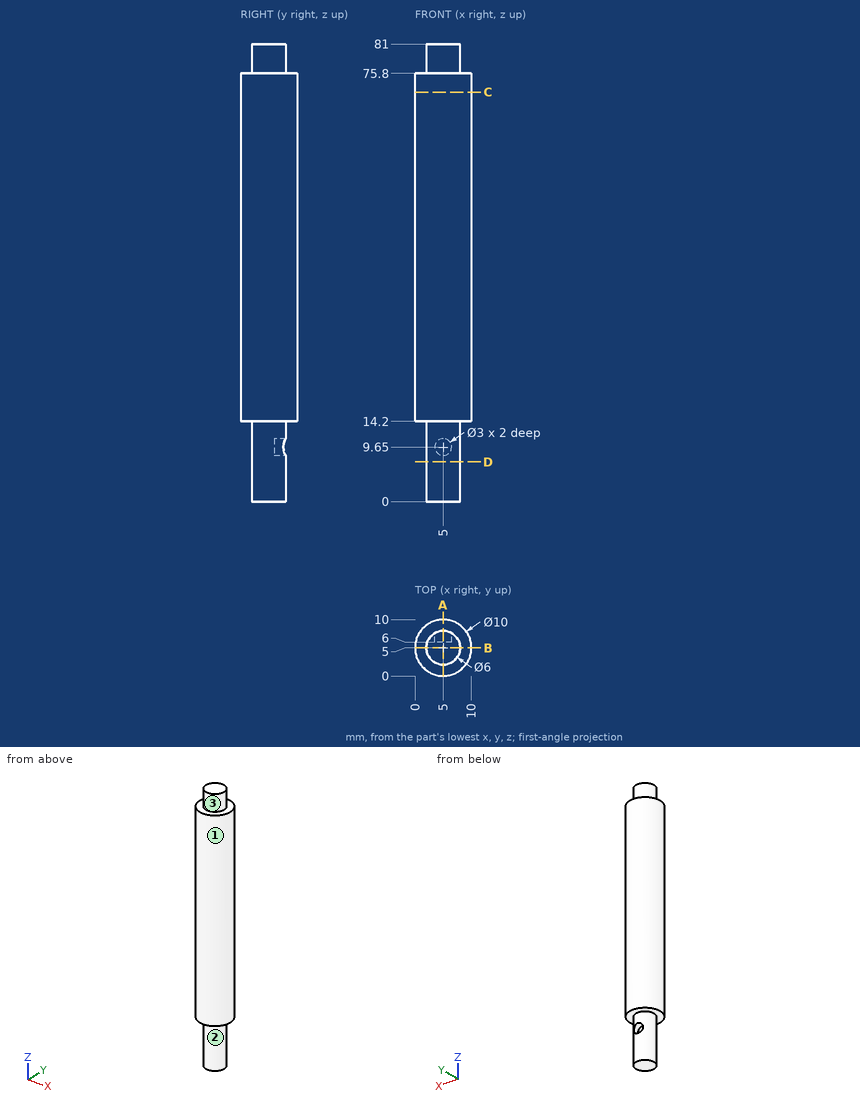
Can you work these out from the drawing? Everything is in mm from the part's minimum corner. A direction names the side the tool comes from. Round coordinates to 2 decimals unless told otherwise and drop trailing zeros. Order: outer loops, then holes, each group sorted by start corner. A loop starts at its lowest first (then second) coordinate and runs counter-clockwise, first axis right, second up. Notation, with made-up numbers: M 21,44 L 26,44 A29 ccw 26,77 Z; hole C 56,65 d9. An arc over 180 degrees is marked long. One line per question, with ' | ' between items.
1) I want a section at C-C, the plane z = 72.5. Write out the boundary of the cut face in (x, y), then the cut area to 3 significant figures.
Working result:
outline: C 5,5 d10 | area: 78.5 mm²
2) I want a section at B-B, the plane y = 5. Write out the boundary of the cut face in (x, z), then the cut area to 3 significant figures.
Working result:
outline: M 0,14.2 L 2,14.2 L 2,0 L 8,0 L 8,14.2 L 10,14.2 L 10,75.8 L 8,75.8 L 8,81 L 2,81 L 2,75.8 L 0,75.8 Z | area: 732 mm²
3) I need wall thicknesses on line 1 along Z through (x, y) = (5, 7.5); line 2 along X through (y, z) = (6.9, 9.65); line 3 along X through (y, z) = (7.2, 9.65). Which ranges of each line are inside material? Lowest first, please.
Working result:
line 1: 0 to 8.15, 11.15 to 81 | line 2: 2.68 to 3.5, 6.5 to 7.32 | line 3: 2.96 to 3.5, 6.5 to 7.04
4) I want a section at A-A, the plane x = 5. Write out the boundary of the cut face in (y, z), then the cut area to 3 significant figures.
Working result:
outline: M 0,14.2 L 2,14.2 L 2,0 L 8,0 L 8,8.15 L 6,8.15 L 6,11.15 L 8,11.15 L 8,14.2 L 10,14.2 L 10,75.8 L 8,75.8 L 8,81 L 2,81 L 2,75.8 L 0,75.8 Z | area: 726 mm²
5) I want a section at D-D, the plane z = 7. Write out the boundary of the cut face in (x, y), then the cut area to 3 significant figures.
Working result:
outline: C 5,5 d6 | area: 28.3 mm²
6) For pin 1 Ø1 at (x, z) = (6, 51.5) entering from +Y; pin 2 Ø5 at (x, z) = (3.5, 24.5) entering from -Y; pin 3 Ø2.5 at (x, z) = (4.5, 10) entering from +Y; pin 4 Ø1 at (y, z) = (6.5, 12.5) entering from -X, each with a flat end and sliding along its axis, tell me the tip position at first contact or that it passes through.
Working result:
pin 1: y = 9.97 | pin 2: y = 0 | pin 3: y = 8 | pin 4: x = 2.17
7) For the marked faces 1, 2 and 3, which set-ups out of +Z, -Z, +X, -X, +Y, -Y let a thin tool reach every point of the face, with its end or its side?
Working result:
face 1: +Z, -Z | face 2: -Z | face 3: +Z
